Verification items for the finished model (mm, model axes). A direction names the side the tool comes from. Give positions to 0.01 mm unless a question says otherwise; leave off trailing zeros. Order: outer loops, then holes, each group sorted by start corner. A loop starts at its lowest first (then second) coordinate and runs counter-clockwise, first axis right, second up. Notation, with made-up numbers: (19, -33.5) - (37, -33.5) arc R32 cw to (37, -1.5) - close; hole circle Ø6 at (28, -39.75). An arc over 180 degrees is marked (long way). Answer as a JSON object with one key per item and string values. Group by question number.
(1) Access from +Z, -Z, +X, -X, +Y, -Y to the whole of each face (thin tool, end or side, straight path). Record for faces 1 (the face through (57, 0, 60)), 2 (the face through (-60, 0, 57)), 3 (the face through (-4.88, 14.93, -1.08)), 4 (the face through (75, -27, -67)).
(2) Section check A-A (y = -65.5). Record the boundary of the cut face in (x, z).
(3) Mould release check, pull along X, two halves, no side actions. Record for faces 5 (the face through (-75, -82, 19)), 6 (the face through (85, -70, 19)), 7 (the face through (-1, -35, -206.035)), 8 (the face through (-85, -70, 19)): +X half, -X half, draft (parallel to the pull), parting line (faces both ways), or undercut.
(4) Depth check by flat-ended pin: pin 1 Ø11.5 at (x, z) = (0, 0) entering from +Y; pin 2 Ø8 at (x, z) = (-22, -14.5) entering from -Y; pin 3 Ø21 at (y, z) = (-51.5, -43.5) entering from +X. Enter the tip coordinate at first touch or a pass-through.
(5) Section check B-B (z = -155.5). Record the boundary of the cut face in (x, y).
(6) Thickness scan on line 1 (X direction, y = 15, z = 0); line 2 (X direction, y = -77, z = 13); line 3 (X direction, y = -7.5, z = 19.5). Record the ranges inside material, lowest first.
```python
from build123d import *

# Parameters (mm, degrees)
SKETCH1_R           = 75
BOSS_EXTRUDE1_DEPTH = 20
FILLET4_R           = 5
CUT_EXTRUDE1_START  = 10
SKETCH2_R           = 5
CUT_EXTRUDE1_DEPTH  = 10
SKETCH3_W           = 150
SKETCH3_H           = 281.035433198
BOSS_EXTRUDE2_DEPTH = 70
SKETCH4_R           = 32.5
BOSS_EXTRUDE3_DEPTH = 10
SKETCH6_R           = 32.5
BOSS_EXTRUDE4_DEPTH = 10
BOSS_EXTRUDE5_START = 10
SKETCH8_R           = 32.5
BOSS_EXTRUDE5_DEPTH = 10
BOSS_EXTRUDE6_START = 10
SKETCH9_R           = 32.5
BOSS_EXTRUDE6_DEPTH = 10
SKETCH10_R          = 3.109945618
BOSS_EXTRUDE7_DEPTH = 80
SKETCH11_R          = 1.721500876
BOSS_EXTRUDE8_DEPTH = 50


with BuildPart() as part:
    # Sketch1 → Boss-Extrude1 (new body)
    with BuildSketch(Plane(origin=(0, 0, 0), x_dir=(1, 0, 0), z_dir=(0, 1, 0))):
        with Locations(Location((0, 0, 0), (0, 0, 270))):
            Circle(SKETCH1_R)
    extrude(amount=BOSS_EXTRUDE1_DEPTH)

    # Fillet4
    fillet4_edges = [part.edges().sort_by_distance(p)[0] for p in [
        (0, 20, -75),
    ]]
    fillet(fillet4_edges, radius=FILLET4_R)

    # Sketch2 → Cut-Extrude1 (cut)
    with BuildSketch(Plane(origin=(0, 0, 0), x_dir=(1, 0, 0), z_dir=(0, 1, 0)).offset(CUT_EXTRUDE1_START)):
        with Locations(Location((0, 0, 0), (0, 0, 270))):
            Circle(SKETCH2_R)
    extrude(amount=CUT_EXTRUDE1_DEPTH, mode=Mode.SUBTRACT)

    # Sketch3 → Boss-Extrude2 (add)
    with BuildSketch(Plane.XZ):
        with Locations((0, -65.517716599)):
            Rectangle(SKETCH3_W, SKETCH3_H)
    extrude(amount=BOSS_EXTRUDE2_DEPTH)

    # Sketch4 → Boss-Extrude3 (add)
    with BuildSketch(Plane.ZY.offset(75)):
        with Locations((-154.802708443, -70)):
            Circle(SKETCH4_R)
    extrude(amount=BOSS_EXTRUDE3_DEPTH)

    # Sketch6 → Boss-Extrude4 (add)
    with BuildSketch(Plane.ZY.offset(75)):
        with Locations((19.016258359, -70)):
            Circle(SKETCH6_R)
    extrude(amount=BOSS_EXTRUDE4_DEPTH)

    # Sketch8 → Boss-Extrude5 (add)
    with BuildSketch(Plane(origin=(75, 0, 0), x_dir=(0, 0, -1), z_dir=(1, 0, 0)).offset(BOSS_EXTRUDE5_START)):
        with Locations(Location((-19.016258359, -70, 0), (0, 0, 180))):
            Circle(SKETCH8_R)
    extrude(amount=-BOSS_EXTRUDE5_DEPTH)

    # Sketch9 → Boss-Extrude6 (add)
    with BuildSketch(Plane(origin=(75, 0, 0), x_dir=(0, 0, -1), z_dir=(1, 0, 0)).offset(BOSS_EXTRUDE6_START)):
        with Locations(Location((154.802708443, -70, 0), (0, 0, 180))):
            Circle(SKETCH9_R)
    extrude(amount=-BOSS_EXTRUDE6_DEPTH)

    # Sketch10 → Boss-Extrude7 (add)
    with BuildSketch(Plane(origin=(0, 0, 0), x_dir=(1, 0, 0), z_dir=(0, 1, 0))):
        with Locations(Location((-56.826635482, 196.658461897, 0), (0, 0, 90))):
            Circle(SKETCH10_R)
    extrude(amount=BOSS_EXTRUDE7_DEPTH)

    # Sketch11 → Boss-Extrude8 (add)
    with BuildSketch(Plane(origin=(0, 0, 0), x_dir=(1, 0, 0), z_dir=(0, 1, 0))):
        with Locations(Location((-48.57774745, 196.85215418, 0), (0, 0, 90))):
            Circle(SKETCH11_R)
    extrude(amount=BOSS_EXTRUDE8_DEPTH)


solid = part.part
```
Solutions:
{
 "1": {"face 1": "+Z, +X, +Y", "face 2": "+Z, -X, +Y", "face 3": "+Y", "face 4": "+X, +Y"},
 "2": {"outline": "(-85, -186.99) - (-75, -186.99) - (-75, -206.04) - (75, -206.04) - (75, -186.99) - (85, -186.99) - (85, -122.62) - (75, -122.62) - (75, -13.17) - (85, -13.17) - (85, 51.2) - (75, 51.2) - (75, 75) - (-75, 75) - (-75, 51.2) - (-85, 51.2) - (-85, -13.17) - (-75, -13.17) - (-75, -122.62) - (-85, -122.62) - close"},
 "3": {"face 5": "undercut", "face 6": "+X half", "face 7": "draft", "face 8": "-X half"},
 "4": {"pin 1": "stops at y = 20", "pin 2": "stops at y = -70", "pin 3": "stops at x = 75"},
 "5": {"outline": "(-85, -102.49) - (-75, -102.49) - (-75, -70) - (75, -70) - (75, -102.49) - (85, -102.49) - (85, -37.51) - (75, -37.51) - (75, 0) - (-75, 0) - (-75, -37.51) - (-85, -37.51) - close"},
 "6": {"line 1": "x = -75 to -5, 5 to 75", "line 2": "x = -85 to -75, 75 to 85", "line 3": "x = -75 to 75"}
}
